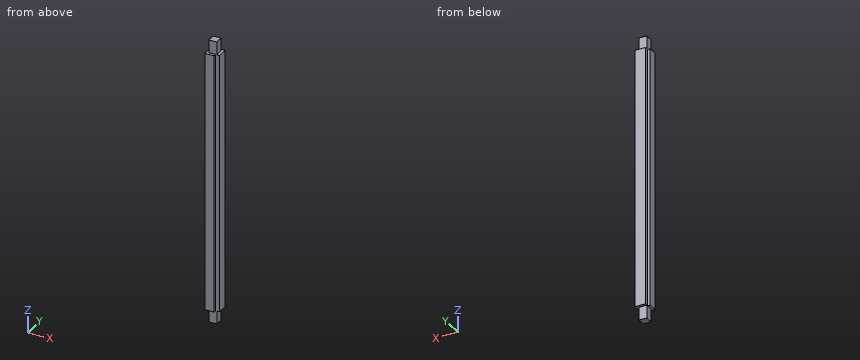
```python
from build123d import *

# Parameters (mm, degrees)
F0_W     = 100
F0_H     = 2200
F1_DEPTH = 100
F2_W     = 30
F2_H     = 2200
F3_DEPTH = 20
F4_W     = 30
F4_H     = 2200
F5_DEPTH = 20
F7_DEPTH = 100
F9_DEPTH = 100


with BuildPart() as f1:
    # F0 (on Front) → F1 (new body)
    with BuildSketch(Plane.XZ):
        with Locations((50, 1100)):
            Rectangle(F0_W, F0_H)
    extrude(amount=F1_DEPTH)

    # F2 (on face) → F3 (cut)
    with BuildSketch(Plane.XZ.offset(100)):
        with Locations((85, 1100)):
            Rectangle(F2_W, F2_H)
    extrude(amount=-F3_DEPTH, mode=Mode.SUBTRACT)

    # F4 (on face) → F5 (cut)
    with BuildSketch(Plane(origin=(0, 0, 0), x_dir=(0, -1, 0), z_dir=(-1, 0, 0))):
        with Locations((15, 1100)):
            Rectangle(F4_W, F4_H)
    extrude(amount=-F5_DEPTH, mode=Mode.SUBTRACT)

    # F6 (on face) → F7 (cut)
    with BuildSketch(Plane.XY.offset(2200)):
        Polygon((20, -20), (80, -20), (80, -80), (100, -80), (100, 0), (20, 0), align=None)
        Polygon((20, -80), (20, -30), (0, -30), (0, -100), (70, -100), (70, -80), align=None)
    extrude(amount=-F7_DEPTH, mode=Mode.SUBTRACT)

    # F8 (on face) → F9 (cut)
    with BuildSketch(Plane(origin=(0, 0, 0), x_dir=(1, 0, 0), z_dir=(0, 0, -1))):
        Polygon((0, 30), (20, 30), (20, 80), (70, 80), (70, 100), (0, 100), align=None)
        Polygon((80, 20), (20, 20), (20, 0), (100, 0), (100, 80), (80, 80), align=None)
    extrude(amount=-F9_DEPTH, mode=Mode.SUBTRACT)


solid = f1.part
```
Geometry: final body of the model. Coordinates: model frame, mm. Round coordinates to 2 decimals unless told otherwise and drop trailing zeros. Loops run counter-clockwise (first coordinate to the right, second up) from the corner with the lowest first, then second, coordinate; pieces in that order, holes last. Notation, with made-up numbers: (37.5, 60.25) -> (70.5, 60.25) arc R20 ccw to (70.5, 78.25) -> close; hole circle Ø4 at (29, 69). An arc over 180 degrees is marked (long way). Write each question's results on one line, items separated by ' | '.
Item 1: Pin query (flat end, axial travel): pin 1 Ø18 at (y, z) = (-44.5, 2165.5) entering from +X; pin 2 Ø6 at (y, z) = (-11.5, 1805) entering from -X; pin 3 Ø10 at (y, z) = (-90, 927) entering from +X. Return the tip coordinate at first contact, or that it passes through.
Answers below:
pin 1: stops at x = 80 | pin 2: stops at x = 20 | pin 3: stops at x = 70
Item 2: Line query: probe 1 along Z at (x, y) = (18.5, -62); probe 2 along Y at (x, z) = (92.5, 788.5); probe 3 along X at (y, z) = (-61, 96). Output: solid intervals per line, ascending. Write a range as [from, to].
Answers below:
probe 1: z = [100, 2100] | probe 2: y = [-80, 0] | probe 3: x = [20, 80]
Item 3: Cut plane C-C on y = -57. Return the cut outline in (x, z).
Answers below:
outline: (0, 100) -> (20, 100) -> (20, 0) -> (80, 0) -> (80, 100) -> (100, 100) -> (100, 2100) -> (80, 2100) -> (80, 2200) -> (20, 2200) -> (20, 2100) -> (0, 2100) -> close
Item 4: Cut plane B-B on x = 48. Return the cut outline in (y, z), and give its area (3 significant figures).
Answers below:
outline: (-100, 100) -> (-80, 100) -> (-80, 0) -> (-20, 0) -> (-20, 100) -> (0, 100) -> (0, 2100) -> (-20, 2100) -> (-20, 2200) -> (-80, 2200) -> (-80, 2100) -> (-100, 2100) -> close | area: 212,000 mm²
Item 5: Cut plane A-A on z = 203.5. Return the cut outline in (x, y).
Answers below:
outline: (0, -100) -> (70, -100) -> (70, -80) -> (100, -80) -> (100, 0) -> (20, 0) -> (20, -30) -> (0, -30) -> close
